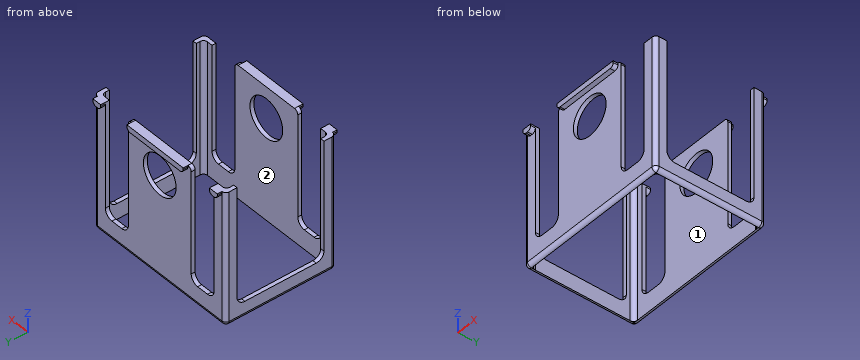
from build123d import *

# Parameters (mm, degrees)
F1_DEPTH  = 170
F2_R      = 25
F3_DEPTH  = 250
F5_DEPTH  = 210
F6_R      = 5
F8_DEPTH  = 6
F9_R      = 4.99999
F11_DEPTH = 6


# Not quite as in the source:
# - a fillet or chamfer is up to 0.001 mm smaller than in the source, because OpenCascade refuses the exact size


with BuildPart() as f1:
    # F0 (on Top) → F1 (new body)
    with BuildSketch(Plane.XY):
        with BuildLine():
            ThreePointArc((100, 65.5), (98.5355339059, 69.0355339059), (95, 70.5))
            Line((95, 70.5), (-95, 70.5))
            ThreePointArc((-95, 70.5), (-98.5355339059, 69.0355339059), (-100, 65.5))
            Line((-100, 65.5), (-100, -65.5))
            ThreePointArc((-100, -65.5), (-98.5355339059, -69.0355339059), (-95, -70.5))
            Line((-95, -70.5), (95, -70.5))
            ThreePointArc((95, -70.5), (98.5355339059, -69.0355339059), (100, -65.5))
            Line((100, -65.5), (100, 65.5))
        make_face()
        with BuildLine():
            Line((-90, 65.5), (90, 65.5))
            ThreePointArc((90, 65.5), (93.5355339059, 64.0355339059), (95, 60.5))
            Line((95, 60.5), (95, -60.5))
            ThreePointArc((95, -60.5), (93.5355339059, -64.0355339059), (90, -65.5))
            Line((90, -65.5), (-90, -65.5))
            ThreePointArc((-90, -65.5), (-93.5355339059, -64.0355339059), (-95, -60.5))
            Line((-95, -60.5), (-95, 60.5))
            ThreePointArc((-95, 60.5), (-93.5355339059, 64.0355339059), (-90, 65.5))
        make_face(mode=Mode.SUBTRACT)
    extrude(amount=F1_DEPTH)

    # F2 (on face) → F3 (cut)
    with BuildSketch(Plane.XZ.offset(70.5)):
        with Locations((0, 130)):
            Circle(F2_R)
        with BuildLine():
            Line((-48, 170), (-83, 170))
            Line((-83, 170), (-83, 35))
            ThreePointArc((-83, 35), (-80.0710678119, 27.9289321881), (-73, 25))
            Line((-73, 25), (-58, 25))
            ThreePointArc((-58, 25), (-50.9289321881, 27.9289321881), (-48, 35))
            Line((-48, 35), (-48, 170))
        make_face()
        with BuildLine():
            Line((83, 170), (48, 170))
            Line((48, 170), (48, 35))
            ThreePointArc((48, 35), (50.9289321881, 27.9289321881), (58, 25))
            Line((58, 25), (73, 25))
            ThreePointArc((73, 25), (80.0710678119, 27.9289321881), (83, 35))
            Line((83, 35), (83, 170))
        make_face()
    extrude(amount=-F3_DEPTH, mode=Mode.SUBTRACT)

    # F4 (on face) → F5 (cut)
    with BuildSketch(Plane.YZ.offset(100)):
        with BuildLine():
            Line((55.5, 170), (-55.5, 170))
            Line((-55.5, 170), (-55.5, 30))
            ThreePointArc((-55.5, 30), (-52.5710678119, 22.9289321881), (-45.5, 20))
            Line((-45.5, 20), (45.5, 20))
            ThreePointArc((45.5, 20), (52.5710678119, 22.9289321881), (55.5, 30))
            Line((55.5, 30), (55.5, 170))
        make_face()
    extrude(amount=-F5_DEPTH, mode=Mode.SUBTRACT)

    # F6
    f6_edges = [f1.edges().sort_by_distance(p)[0] for p in [
        (-48, -68, 170),
        (48, -68, 170),
        (48, 68, 170),
        (-48, 68, 170),
    ]]
    fillet(f6_edges, radius=F6_R)

    # F7 (on face) → F8 (join)
    with BuildSketch(Plane.XZ.offset(70.5)):
        with BuildLine():
            ThreePointArc((-88, 163), (-84.4644660941, 164.4644660941), (-83, 168))
            Line((-83, 168), (-83, 170))
            Line((-83, 170), (-95, 170))
            Line((-95, 170), (-95, 167.7))
            ThreePointArc((-95, 167.7), (-93.6234018716, 164.3765981284), (-90.3, 163))
            Line((-90.3, 163), (-88, 163))
        make_face()
        with BuildLine():
            Line((43, 170), (-43, 170))
            Line((-43, 170), (-43, 167.7))
            ThreePointArc((-43, 167.7), (-41.6234018716, 164.3765981284), (-38.3, 163))
            Line((-38.3, 163), (38.3, 163))
            ThreePointArc((38.3, 163), (41.6234018716, 164.3765981284), (43, 167.7))
            Line((43, 167.7), (43, 170))
        make_face()
    extrude(amount=F8_DEPTH)

    # F9 (radius 5 in the source; OpenCascade refuses exactly that, so slightly less here)
    f9_edges = [f1.edges().sort_by_distance(p)[0] for p in [
        (-100, 0, 0),
    ]]
    fillet(f9_edges, radius=F9_R)

    # F10 (on face) → F11 (join)
    with BuildSketch(Plane(origin=(0, 70.5, 0), x_dir=(-1, 0, 0), z_dir=(0, 1, 0))):
        with BuildLine():
            ThreePointArc((-88, 163), (-84.4644660941, 164.4644660941), (-83, 168))
            Line((-83, 168), (-83, 170))
            Line((-83, 170), (-95, 170))
            Line((-95, 170), (-95, 168))
            ThreePointArc((-95, 168), (-93.5355339059, 164.4644660941), (-90, 163))
            Line((-90, 163), (-88, 163))
        make_face()
        with BuildLine():
            Line((43, 170), (-43, 170))
            Line((-43, 170), (-43, 168))
            ThreePointArc((-43, 168), (-41.5355339059, 164.4644660941), (-38, 163))
            Line((-38, 163), (38, 163))
            ThreePointArc((38, 163), (41.5355339059, 164.4644660941), (43, 168))
            Line((43, 168), (43, 170))
        make_face()
        with BuildLine():
            Line((83, 170), (83, 168))
            ThreePointArc((83, 168), (84.4644660941, 164.4644660941), (88, 163))
            Line((88, 163), (90, 163))
            ThreePointArc((90, 163), (93.5355339059, 164.4644660941), (95, 168))
            Line((95, 168), (95, 170))
            Line((95, 170), (83, 170))
        make_face()
    extrude(amount=F11_DEPTH)


solid = f1.part
The listing builds one solid part. Answer for the finished solid, in the listing's coordinates (mm). Face numbers are marked on the shaded views. Coordinates: 2 decimals unless noted, no trailing zeros. Use CSV: the item, a comma, the result in double quotes.
Q1. Straight lines are drawn through the part: L1, parallel to Y at x = 20, z = 7.5; L2, parallel to X at y = -63.5, z = 113; L3, parallel to Z at x = 0, y = 66.6. For each, find the intervals that lie inside material, in ascending order.
Here are the results:
L1,"-70.5 to -65.5, 65.5 to 70.5"
L2,"-100 to -94, 94 to 100"
L3,"0.12 to 105, 155 to 170"
Q2. Determine the mould class of the marked faces 1 and 2 for opening direction X: pulls with the +X half, pulls with the -X half, needs draft (parallel to the pull), parting line crosses it, or undercut.
Here are the results:
face 1,"undercut"
face 2,"undercut"
Q3. Section A-A (x = 0) is taken. Give the number of separate pieces and of enclosed holes in the cut face, then the cut area to 3 significant figures.
Here are the results:
separate pieces,"4"
enclosed holes,"0"
area,"1,270 mm2"
Q4. Given pin 1 Ø2.5 at (x, y) = (-89, -72.5) entering from -Z; pin 2 Ø5.5 at (x, y) = (-66.5, -69) entering from +Z; pin 3 Ø1.5 at (x, z) = (-96.5, 88) entering from +Y; pin 4 Ø5.5 at (y, z) = (67, 79.5) entering from -X, each flat-ended and moving along its own axis, determine where each tip first touches the part or whether it passes through.
Here are the results:
pin 1,"z = 163"
pin 2,"z = 25"
pin 3,"y = 70.44"
pin 4,"x = -100"
